Could you check a few things on this model? Use its own coordinates, in mm. Face numbers are marked on the shaded views. A direction names the side the tool comes from. Coordinates: 2 decimals unless noted, no trailing zeros. Loops run counter-clockwise (first coordinate to the right, second up) from the corner with the lowest first, then second, coordinate; pieces in that order, holes last.
from build123d import *

# Parameters (mm, degrees)
SKETCH1_W               = 140.9
SKETCH1_H               = 204
BOSS_EXTRUDE1_DEPTH     = 4
SKETCH4_W               = 140.9
SKETCH4_H               = 6
BOSS_EXTRUDE3_DEPTH     = 22
CUT_EXTRUDE1_DEPTH      = 217.940550612
CUT_EXTRUDE1_DEPTH_BACK = 217.940550612
SKETCH5_R               = 2
CUT_EXTRUDE4_DEPTH      = 4
SKETCH9_R               = 2
CUT_EXTRUDE5_DEPTH      = 212.308311479
CUT_EXTRUDE6_DEPTH      = 4
CHAMFER1_SIZE           = 0.5


with BuildPart() as part:
    # Sketch1 → Boss-Extrude1 (new body)
    with BuildSketch(Plane.XY):
        Rectangle(SKETCH1_W, SKETCH1_H)
    extrude(amount=-BOSS_EXTRUDE1_DEPTH)

    # Sketch4 → Boss-Extrude3 (add)
    with BuildSketch(Plane.XY):
        with Locations((0, 99)):
            Rectangle(SKETCH4_W, SKETCH4_H)
        with Locations((0, -99)):
            Rectangle(SKETCH4_W, SKETCH4_H)
    extrude(amount=BOSS_EXTRUDE3_DEPTH)

    # Sketch5 → Cut-Extrude1 (cut, two sides: drawn at the far end of the back side and taken through both)
    with BuildSketch(Plane(origin=(0, 102, 0), x_dir=(1, 0, 0), z_dir=(0, 1, 0)).offset(-CUT_EXTRUDE1_DEPTH_BACK)):
        with Locations(Location((-30, -8, 0), (0, 0, 270))):
            Circle(SKETCH5_R)
        with Locations(Location((-60, -8, 0), (0, 0, 270))):
            Circle(SKETCH5_R)
        with Locations(Location((60, -8, 0), (0, 0, 90))):
            Circle(SKETCH5_R)
        with Locations(Location((30, -8, 0), (0, 0, 90))):
            Circle(SKETCH5_R)
    extrude(amount=CUT_EXTRUDE1_DEPTH + CUT_EXTRUDE1_DEPTH_BACK, mode=Mode.SUBTRACT)

    # Sketch8 → Cut-Extrude4 (cut)
    with BuildSketch(Plane(origin=(0, -96, 0), x_dir=(1, 0, 0), z_dir=(0, 1, 0))):
        Polygon((-26.016283143, -8), (-28.008141571, -4.55), (-31.991858429, -4.55), (-33.983716857, -8), (-31.991858429, -11.45), (-28.008141571, -11.45), align=None)
        Polygon((-56.016283143, -8), (-58.008141571, -4.55), (-61.991858429, -4.55), (-63.983716857, -8), (-61.991858429, -11.45), (-58.008141571, -11.45), align=None)
        Polygon((33.983716857, -8), (31.991858429, -4.55), (28.008141571, -4.55), (26.016283143, -8), (28.008141571, -11.45), (31.991858429, -11.45), align=None)
        Polygon((63.983716857, -8), (61.991858429, -4.55), (58.008141571, -4.55), (56.016283143, -8), (58.008141571, -11.45), (61.991858429, -11.45), align=None)
    cut_extrude4 = extrude(amount=-CUT_EXTRUDE4_DEPTH, mode=Mode.SUBTRACT)

    # Mirror1: Cut-Extrude4 across plane
    add(cut_extrude4.mirror(Plane.ZX), mode=Mode.SUBTRACT)

    # Sketch9 → Cut-Extrude5 (cut, through all)
    with BuildSketch(Plane(origin=(0, -96, 0), x_dir=(1, 0, 0), z_dir=(0, 1, 0))):
        with Locations(Location((0, -8, 0), (0, 0, 270))):
            Circle(SKETCH9_R)
    extrude(amount=-CUT_EXTRUDE5_DEPTH, mode=Mode.SUBTRACT)

    # Sketch10 → Cut-Extrude6 (cut)
    with BuildSketch(Plane(origin=(0, -96, 0), x_dir=(1, 0, 0), z_dir=(0, 1, 0))):
        Polygon((1.991858429, -4.55), (-1.991858429, -4.55), (-3.983716857, -8), (-1.991858429, -11.45), (1.991858429, -11.45), (3.983716857, -8), align=None)
    extrude(amount=-CUT_EXTRUDE6_DEPTH, mode=Mode.SUBTRACT)

    # Chamfer1
    chamfer1_edges = [part.edges().sort_by_distance(p)[0] for p in [
        (32.987787643, -96, 9.725),
        (32.987787643, -96, 6.275),
        (30, -96, 4.55),
        (27.012212357, -96, 6.275),
        (27.012212357, -96, 9.725),
        (30, -96, 11.45),
        (62.987787643, -96, 9.725),
        (62.987787643, -96, 6.275),
        (60, -96, 4.55),
        (57.012212357, -96, 6.275),
        (57.012212357, -96, 9.725),
        (60, -96, 11.45),
        (-57.012212357, 96, 9.725),
        (-57.012212357, 96, 6.275),
        (-60, 96, 4.55),
        (-62.987787643, 96, 6.275),
        (-62.987787643, 96, 9.725),
        (-60, 96, 11.45),
        (-27.012212357, 96, 9.725),
        (-27.012212357, 96, 6.275),
        (-30, 96, 4.55),
        (-32.987787643, 96, 6.275),
        (-32.987787643, 96, 9.725),
        (-30, 96, 11.45),
        (32.987787643, 96, 9.725),
        (32.987787643, 96, 6.275),
        (30, 96, 4.55),
        (27.012212357, 96, 6.275),
        (27.012212357, 96, 9.725),
        (30, 96, 11.45),
        (62.987787643, 96, 9.725),
        (62.987787643, 96, 6.275),
        (60, 96, 4.55),
        (57.012212357, 96, 6.275),
        (57.012212357, 96, 9.725),
        (60, 96, 11.45),
        (2.987787643, -96, 6.275),
        (0, -96, 4.55),
        (-2.987787643, -96, 6.275),
        (-2.987787643, -96, 9.725),
        (0, -96, 11.45),
        (2.987787643, -96, 9.725),
        (-57.012212357, -96, 9.725),
        (-57.012212357, -96, 6.275),
        (-60, -96, 4.55),
        (-62.987787643, -96, 6.275),
        (-62.987787643, -96, 9.725),
        (-60, -96, 11.45),
        (-27.012212357, -96, 9.725),
        (-27.012212357, -96, 6.275),
        (-30, -96, 4.55),
        (-32.987787643, -96, 6.275),
        (-32.987787643, -96, 9.725),
        (-30, -96, 11.45),
    ]]
    chamfer(chamfer1_edges, length=CHAMFER1_SIZE)


solid = part.part
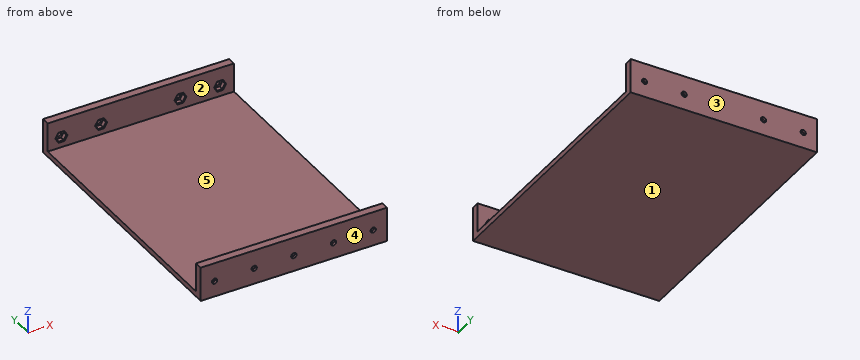
(1) Which directions (+Z, -Z, +X, -X, +Y, -Y) give clear straight access to the entire face, cutting with the end or side of a thin tool? Please do the marked faces 4 and 5.
Answers:
face 4: +Z, -Z, +X, -X, -Y
face 5: +Z, +X, -X
(2) For pin 1 (4.5 mm diameter, centred on x = 30, z = 8, fed in from -Y); pin 2 (8 mm diameter, centred on x = -14, y = -13, fed in from +Z), each with a flat end and sliding along its axis, tell me the tip position at first contact or that it passes through.
Answers:
pin 1: stops at y = -102
pin 2: stops at z = 0
(3) We'd pull the mould along Y, two halves only. Please class the marked faces 1, 2 and 3: +Y half, -Y half, draft (parallel to the pull), parting line (faces both ways), or undercut.
Answers:
face 1: draft
face 2: undercut
face 3: +Y half
(4) Imagine slicing it at B-B, the plane y = 53. Write out the boundary of the cut face in (x, z), and give its area (3 significant figures).
Answers:
outline: (-70.45, -4) - (70.45, -4) - (70.45, 0) - (-70.45, 0) - close
area: 564 mm2
(5) I need wall thicknesses on probe 1 along X at (y, z) = (-101.2, 8); probe 2 along X at (y, z) = (101.35, 8); probe 3 along Y at (x, z) = (38.5, 19.75). Which ranges of each line are inside material? Lowest first, please.
Answers:
probe 1: x = -70.45 to -62, -58 to -32, -28 to -2, 2 to 28, 32 to 58, 62 to 70.45
probe 2: x = -70.45 to -62, -58 to -32, -28 to 28, 32 to 58, 62 to 70.45
probe 3: y = -102 to -96, 96 to 102
(6) Imagine slicing it at A-A, the plane x = 39. Write out the boundary of the cut face in (y, z).
Answers:
outline: (-102, -4) - (102, -4) - (102, 22) - (96, 22) - (96, 0) - (-96, 0) - (-96, 22) - (-102, 22) - close
